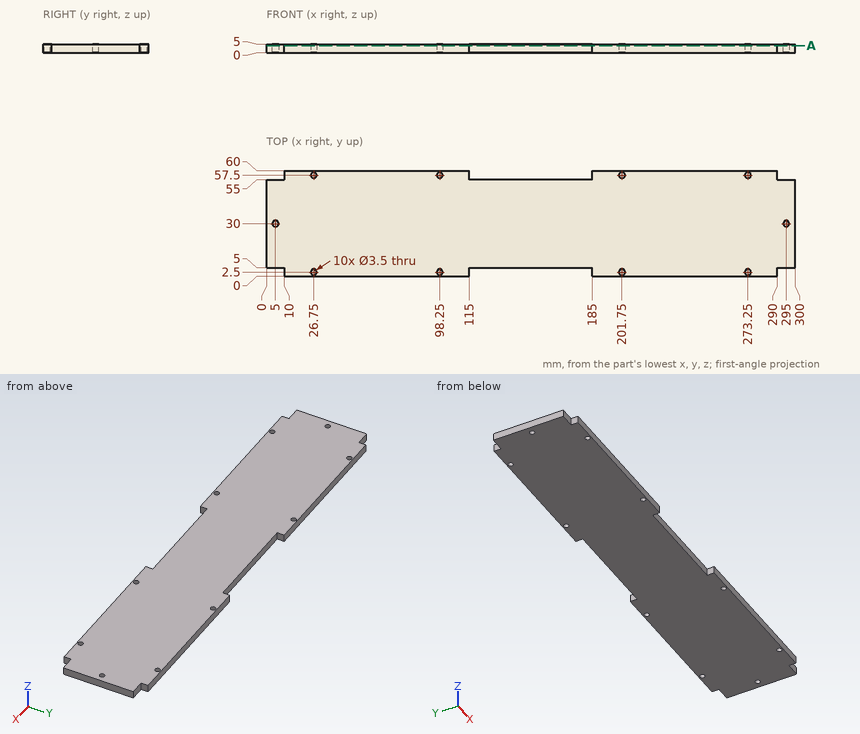
For this review, use the dimensioned drawing (mm, ordinates from the lowest corner) and the shaded views. Give positions to 0.01 mm unless a question says otherwise; leave off trailing zeros.
1) Insertion check: pin 1 (1.5 mm diameter, centred on x = 296.5, z = 3.5, fed in from -Y); pin 2 (1.5 mm diameter, centred on y = 58, z = 1.5, fed in from +X); pin 3 (2 mm diameter, centred on x = 98.25, y = 2.5, fed in from -Z). Each pin has a flat end and moves straight along its axis. Give the tip position at first contact, or say it passes through.
2) Wall thickness on line 1 (Y direction, x = 201.75, z = 4.05); line 2 (Y direction, x = 295, z = 3.8); line 3 (Y direction, x = 140, z = 3.55): over which ranges is each line inside the solid? List them lowest first.
3) Take a section at A-A (z = 4.1). State how many separate pieces and enclosed holes the cut face has, then the cut area to 3 significant figures.
Derived:
1. pin 1: stops at y = 5
1. pin 2: stops at x = 290
1. pin 3: passes through
2. line 1: y = 0 to 0.75, 4.25 to 55.75, 59.25 to 60
2. line 2: y = 5 to 28.25, 31.75 to 55
2. line 3: y = 5 to 55
3. separate pieces: 1
3. enclosed holes: 10
3. area: 17,000 mm2
